Autodesk Inventor part; units mm, degrees
ref_plane "YZ Plane" through (0, 0, 0) normal (1, 0, 0) x (0, 1, 0)
ref_plane "XZ Plane" through (0, 0, 0) normal (0, 1, 0) x (-1, 0, 0)
ref_plane "XY Plane" through (0, 0, 0) normal (0, 0, 1) x (1, 0, 0)
sketch "Sketch3" plane through (0, 0, 0) normal (0, 0, 1) x (1, 0, 0)
  circle A0 centre (0, 0) radius 4.45
  dimension "d11" = 8.9
extrude "Extrusion3" add sketch "Sketch3" along normal blind 6
sketch "Sketch4" plane through (0, 0, 6) normal (0, 0, 1) x (1, 0, 0)
  circle A0 centre (0, 0) radius 30
  dimension "d14" = 60
extrude "Extrusion4" add sketch "Sketch4" along normal blind 8
ref_plane "Work Plane2" through (0, 0, 8) normal (0, 0, 1) x (1, 0, 0)
ref_plane "Work Plane1" through (0, 0, 10) normal (0, 0, 1) x (1, 0, 0)
sketch "Sketch5" plane through (0, 0, 8) normal (0, 0, 1) x (1, 0, 0)
  arc A0 (0.5639, -28.4944) -> (-0.5169, -28.4953) centre (0, 0) ccw
  circle A1 centre (0, 0) radius 30
  line L0 (0.5639, -28.4944) -> (0.5639, -23.859)
  line L1 (0.5639, -23.859) -> (-0.5169, -23.859)
  line L2 (-0.5169, -23.859) -> (-0.5169, -28.4953)
  dimension "d17" = 57
  dimension "d18" = 60
extrude "Extrusion5" cut sketch "Sketch5" along normal mid plane 2
mirror "Mirror1" about plane through (0, 0, 10) normal (0, 0, 1) of "Extrusion5"
sketch "Sketch9" plane through (0, 0, 0) normal (0, 0, -1) x (-1, 0, 0)
  circle A0 centre (0, 0) radius 4.45
  circle A1 centre (0, 0) radius 4.45
  dimension "d40" = 8.9
extrude "Extrusion9" cut sketch "Sketch9" against normal blind 6
sketch "Sketch10" plane through (0, 0, 14) normal (0, 0, 1) x (1, 0, 0)
  circle A0 centre (0, -28.6156) radius 0.75
  point P0 (0, 0)
  dimension "d43" = 1.5
extrude "Extrusion10" cut sketch "Sketch10" against normal blind 10
sketch "Sketch11" plane through (0, 0, 14) normal (0, 0, 1) x (1, 0, 0)
  line L0 (1.9614, -3.4009) -> (-1.9645, -3.3991)
  line L1 (-1.9645, -3.3991) -> (-3.926, 0.0018)
  line L2 (-3.926, 0.0018) -> (-1.9614, 3.4009)
  line L3 (-1.9614, 3.4009) -> (1.9645, 3.3991)
  line L4 (1.9645, 3.3991) -> (3.926, -0.0018)
  line L5 (3.926, -0.0018) -> (1.9614, -3.4009)
  point P0 (0, 0)
  point P1 (0, 0)
  dimension "d46" = 6.8
extrude "Extrusion11" cut sketch "Sketch11" against normal blind 10
ref_plane "Work Plane3" through (0, 0, 10) normal (0, 0, 1) x (1, 0, 0)
ref_plane "Work Plane4" through (0, 0, 12) normal (0, 0, 1) x (1, 0, 0)
properties part number "PulleyWithHole" material "ABS Plastic"
Geometry: final body of the model. Coordinates: model frame, mm. A direction names the side the tool comes from. Coordinates: 2 decimals unless noted, no trailing zeros. Loops run counter-clockwise (first coordinate to the right, second up) from the corner with the lowest first, then second, coordinate; pieces in that order, holes last. Notation, with made-up numbers: M 26.25,-5.75 L 47.25,-5.75 A24 cw 47.25,20.25 Z; hole C -38,-12 d5. An arc over 180 degrees is marked long. One line per item, written item: value. Start each with the question number.
1) Cut plane B-B (y = -10.5). Return loops of the section in (x, z), then the cut area to 3 significant figures.
2) Cut plane A-A (x = -21). Return loops of the section in (y, z).
3) Pin query (flat end, axial travel): P1, Ø0.5, axis at x = 0, z = 12, coming from the -Y side; P2, Ø2, axis at x = -8.5, z = 11.5, coming from the -Y side; P3, Ø0.6, axis at y = -25, z = 8.5, coming from the -X side. Return the tip coordinate at first contact, or that it passes through.
4) Reachability of faces 4 (the flat face through (2.957, -1.678, 10.056)), 5 (the flat face through (-0.517, -26, 12)), 6 (the flat face through (-27, -11, 11)), 7 (the flat face through (0, -6, 14)) from +Z, -Z, +X, -X, +Y, -Y: full face, straight path, thin tool, end or side. Return the list, or none.
5) Draft query along Y for faces 1 (the flat face through (0, -6, 6)), 2 (the cylindrical face through (1.242, 28.473, 12.014)), 3 (the cylindrical face through (0.4, -27.98, 10.06)). Return one class per face: released by +Y, released by -Y, zero draft, split by the parting line, or undercut.
6) Material intervals for L1, parallel to Y at x = 0, z = 10.75; L2, parallel to Y at x = 0, z = 8.5; L3, parallel to Y at x = -1, z = 9.5, sorted ascending. Write a range as from..to.
Evaluation:
1. outline: M -28.1,6 L 28.1,6 L 28.1,7 L 26.5,7 L 26.5,9 L 28.1,9 L 28.1,11 L 26.5,11 L 26.5,13 L 28.1,13 L 28.1,14 L -28.1,14 L -28.1,13 L -26.5,13 L -26.5,11 L -28.1,11 L -28.1,9 L -26.5,9 L -26.5,7 L -28.1,7 Z
1. area: 437 mm^2
2. outline: M -21.42,6 L 21.42,6 L 21.42,7 L 19.27,7 L 19.27,9 L 21.42,9 L 21.42,11 L 19.27,11 L 19.27,13 L 21.42,13 L 21.42,14 L -21.42,14 L -21.42,13 L -19.27,13 L -19.27,11 L -21.42,11 L -21.42,9 L -19.27,9 L -19.27,7 L -21.42,7 Z
3. P1: y = -23.86
3. P2: y = -29.01
3. P3: x = -14.22
4. face 4: +Z, -Z
4. face 5: -Y
4. face 6: none
4. face 7: +Z, +X, -X, +Y, -Y
5. face 1: zero draft
5. face 2: split by the parting line
5. face 3: undercut
6. L1: -30..-29.37, -27.87..-3.4, 3.4..30
6. L2: -23.86..-3.4, 3.4..28.5
6. L3: -29.98..-3.4, 3.4..29.98
